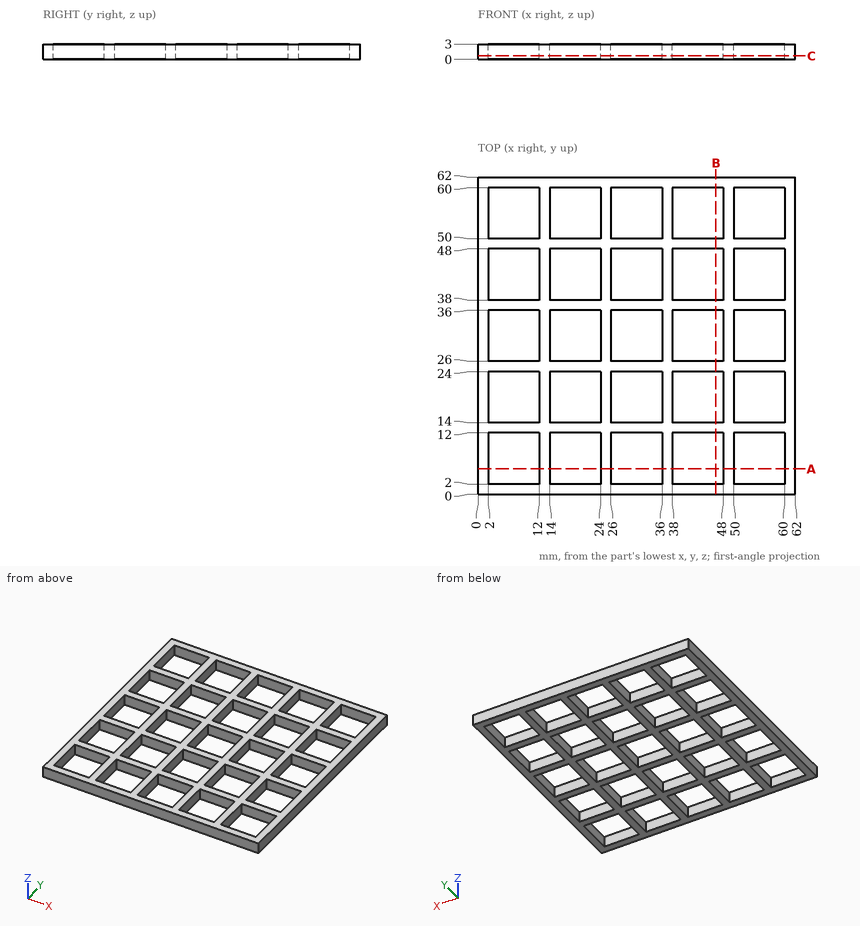
Source: three-view drawing plus pictorial views. Frame: mm from the lowest corner of the part. Round coordinates to 2 decimals unless told otherwise and drop trailing zeros. Loops run counter-clockwise (first coordinate to the right, second up) from the corner with the lowest first, then second, coordinate; pieces in that order, holes last. Notation, with made-up numbers: (-6, 10.5) - (16, 10.5) arc R13 ccw to (16, 21.5) - close; hole circle Ø6 at (82, 18). An arc over 180 degrees is marked (long way). Write each question's results on one line, items separated by ' | '. Start each with the question number.
1) Cut plane A-A on y = 5. Return loops of the section in (x, z), then the cut area to 3 significant figures.
2) First-contact query: P1, Ø2, axis at x = 42.5, y = 40, coming from the +Z side. Flat tip, straight axial feed; report the tip coordinate or a pass-through.
3) Cut plane C-C on z = 0.7. Count the separate pieces of the cut face and the enclosed holes in it, then the cut area to 3 significant figures.
4) Line query: probe 1 along X at (y, z) = (33, 2.4). Output: solid intervals per line, ascending. Write a range as [from, to].
Verdict:
1) outline: (0, 0) - (2, 0) - (2, 3) - (0, 3) - close; (12, 0) - (14, 0) - (14, 3) - (12, 3) - close; (24, 0) - (26, 0) - (26, 3) - (24, 3) - close; (36, 0) - (38, 0) - (38, 3) - (36, 3) - close; (48, 0) - (50, 0) - (50, 3) - (48, 3) - close; (60, 0) - (62, 0) - (62, 3) - (60, 3) - close | area: 36.0 mm2
2) P1: passes through
3) separate pieces: 1 | enclosed holes: 25 | area: 1,340 mm2
4) probe 1: x = [0, 2], [12, 14], [24, 26], [36, 38], [48, 50], [60, 62]
